Build history of the part. All positions in model axes, mm. Round coordinates to 2 decimals unless told otherwise and drop trailing zeros. Write each loop counter-clockwise with the first axis right and the second up, starting at its lowest first coordinate (ties: lowest second). Pieces come first, ordered by that corner, then holes. Notation, with made-up numbers: (27.25, 62) - (41.25, 62) arc R21 ccw to (41.25, 87) - close; hole circle Ø6 at (69.5, -23.75). An arc over 180 degrees is marked (long way). Answer as a JSON object with one key per item and string values. Group by question number.
Item 1: Probe line 1 (X direction, y = 0.4, z = -17) (3 decimals); line 2 (X direction, y = 0.7, z = 24.5). List the from-to ranges inside material, lowest first. Write a range as from..to.
Item 2: Slice it at B-B, the plane z = -8. List the corners of the cut face in (x, y) (3 decimals), then the cut area to 3 significant figures.
Item 3: Slice it at A-A, the plane y = 0.15. List the corners of the cut face in (x, z) (3 decimals), then the cut area to 3 significant figures.
Autodesk Inventor part; units mm, degrees
ref_plane "YZ Plane" through (0, 0, 0) normal (1, 0, 0) x (0, 1, 0)
ref_plane "XZ Plane" through (0, 0, 0) normal (0, 1, 0) x (-1, 0, 0)
ref_plane "XY Plane" through (0, 0, 0) normal (0, 0, 1) x (1, 0, 0)
sketch "Sketch1" plane through (0, 0, 0) normal (0, 1, 0) x (-1, 0, 0)
  line L0 (42.8, -26.99) -> (-42.8, -26.99)
  line L1 (-42.8, -26.99) -> (-42.8, 26.99)
  line L2 (-42.8, 26.99) -> (42.8, 26.99)
  line L3 (42.8, 26.99) -> (42.8, -26.99)
  line L4 (42.8, -26.99) -> (-42.8, 26.99) construction
  line L5 (-42.8, -26.99) -> (42.8, 26.99) construction
  point P0 (0, 0)
  dimension "d0" = 85.6
  dimension "d1" = 53.98
extrude "Extrusion1" add sketch "Sketch1" along normal blind 0.76
fillet "Fillet1" radius 2.88 4 edges at (42.8, 0.38, 26.99) (42.8, 0.38, -26.99) (-42.8, 0.38, 26.99) (-42.8, 0.38, -26.99)
sketch "Sketch2" plane through (0, 0, 0) normal (0, -1, 0) x (1, 0, 0)
  arc A0 (-42.8, -24.11) -> (-39.92, -26.99) centre (-39.92, -24.11) ccw
  line L0 (-39.92, -26.99) -> (39.92, -26.99)
  arc A1 (39.92, -26.99) -> (42.8, -24.11) centre (39.92, -24.11) ccw
  line L1 (42.8, -24.11) -> (42.8, 24.11)
  arc A2 (42.8, 24.11) -> (39.92, 26.99) centre (39.92, 24.11) ccw
  line L2 (39.92, 26.99) -> (-39.92, 26.99)
  arc A3 (-39.92, 26.99) -> (-42.8, 24.11) centre (-39.92, 24.11) ccw
  line L3 (-42.8, 24.11) -> (-42.8, -24.11)
  line L4 (-42.8, 24.11) -> (-42.8, -24.11)
  line L5 (-42.8, -3.99) -> (-39.625, -3.99)
  line L6 (-39.625, -3.99) -> (-39.625, -23.99)
  line L7 (-39.625, -23.99) -> (-42.8, -23.99)
  line L8 (-42.8, -23.99) -> (-42.8, -3.99)
  line L9 (42.8, 24.11) -> (42.8, -24.11)
  line L10 (42.8, -23.99) -> (39.625, -23.99)
  line L11 (39.625, -23.99) -> (39.625, -3.99)
  line L12 (39.625, -3.99) -> (42.8, -3.99)
  line L13 (42.8, -3.99) -> (42.8, -23.99)
  point P0 (0, 0)
  dimension "d5" = 3.175
  dimension "d6" = 3.175
  dimension "d7" = 3
  dimension "d8" = 3
  dimension "d9" = 20
  dimension "d10" = 20
extrude "Extrusion2" cut sketch "Sketch2" against normal through all contours L3 L5 L6 L7 | L10 L11 L12 L1
sketch "Sketch3" plane through (42.8, 0, 24.11) normal (1, 0, 0) x (0, 0, -1)
  line L0 (51.1, 0) -> (51.1, 0.76)
  line L1 (51.1, 0) -> (51.1, 0.76)
  line L2 (48.1, 0.76) -> (48.1, 0)
  line L3 (48.1, 0) -> (51.1, 0.76) construction
  line L4 (51.1, 0) -> (48.1, 0.76) construction
  line L5 (51.1, 0) -> (48.22, 0)
  arc A0 (48.1489, 0.76) -> (48.1489, 0) centre (49.6, 0.38) ccw
  arc A1 (51.0511, 0) -> (51.0511, 0.76) centre (49.6, 0.38) ccw
  line L6 (48.1, 0) -> (48.1489, 0)
  line L7 (51.0511, 0) -> (51.1, 0)
  line L8 (51.1, 0.76) -> (51.0511, 0.76)
  line L9 (48.1489, 0.76) -> (48.1, 0.76)
  point P0 (24.11, 0)
  point P1 (48.1, 0.38)
  point P2 (51.1, 0.38)
  dimension "d14" = 3
  dimension "d15" = 0.76
  dimension "d16" = 1.5
  dimension "d17" = 1.5
  dimension "d18" = 1.5
extrude "Extrusion3" cut sketch "Sketch3" against normal up to surface (3.175 mm away)
mirror "Mirror1" about plane through (0, 0, 0) normal (1, 0, 0) of "Extrusion3"
sketch "Sketch4" plane through (0, 0, 0) normal (0, -1, 0) x (1, 0, 0)
  line L0 (-39.625, -24.0389) -> (-42.8, -24.0389)
  line L1 (-42.8, -24.0389) -> (-42.8, -24.11)
  arc A0 (-42.8, -24.11) -> (-40.4486, -26.9411) centre (-39.92, -24.11) ccw
  line L2 (-40.4486, -26.9411) -> (-39.625, -26.9411)
  line L3 (-39.625, -26.9411) -> (-39.625, -26.99)
  line L4 (-39.625, -26.99) -> (39.625, -26.99)
  line L5 (39.625, -26.99) -> (39.625, -26.9411)
  line L6 (39.625, -26.9411) -> (40.4486, -26.9411)
  arc A1 (40.4486, -26.9411) -> (42.8, -24.11) centre (39.92, -24.11) ccw
  line L7 (42.8, -24.11) -> (42.8, -24.0389)
  line L8 (42.8, -24.0389) -> (39.625, -24.0389)
  line L9 (39.625, -24.0389) -> (39.625, -3.99)
  line L10 (39.625, -3.99) -> (42.8, -3.99)
  line L11 (42.8, -3.99) -> (42.8, 24.11)
  arc A2 (42.8, 24.11) -> (39.92, 26.99) centre (39.92, 24.11) ccw
  line L12 (39.92, 26.99) -> (-39.92, 26.99)
  arc A3 (-39.92, 26.99) -> (-42.8, 24.11) centre (-39.92, 24.11) ccw
  line L13 (-42.8, 24.11) -> (-42.8, -3.99)
  line L14 (-42.8, -3.99) -> (-39.625, -3.99)
  line L15 (-39.625, -3.99) -> (-39.625, -24.0389)
  line L16 (39.92, 26.99) -> (-39.92, 26.99)
  line L17 (42.8, -3.99) -> (42.8, 24.11)
  line L18 (-42.8, 24.11) -> (-42.8, -3.99)
  line L19 (-42.8, 26.99) -> (42.8, 26.99) construction
  line L20 (42.8, 26.99) -> (42.8, -27.0263) construction
  line L21 (42.8, -27.0263) -> (-42.8, -27.0263) construction
  line L22 (-42.8, -27.0263) -> (-42.8, 26.99) construction
  point P0 (0, 0)
decal "Decal1"
sketch "Sketch5" plane through (0, 0.76, 0) normal (0, 1, 0) x (1, 0, 0)
  line L0 (-42.8, 24.0389) -> (-39.625, 24.0389)
  line L1 (-39.625, 24.0389) -> (-39.625, 3.99)
  line L2 (-39.625, 3.99) -> (-42.8, 3.99)
  line L3 (-42.8, 3.99) -> (-42.8, -24.11)
  arc A0 (-42.8, -24.11) -> (-39.92, -26.99) centre (-39.92, -24.11) ccw
  line L4 (-39.92, -26.99) -> (39.92, -26.99)
  arc A1 (39.92, -26.99) -> (42.8, -24.11) centre (39.92, -24.11) ccw
  line L5 (42.8, -24.11) -> (42.8, 3.99)
  line L6 (42.8, 3.99) -> (39.625, 3.99)
  line L7 (39.625, 3.99) -> (39.625, 24.0389)
  line L8 (39.625, 24.0389) -> (42.8, 24.0389)
  line L9 (42.8, 24.0389) -> (42.8, 24.11)
  arc A2 (42.8, 24.11) -> (40.4486, 26.9411) centre (39.92, 24.11) ccw
  line L10 (40.4486, 26.9411) -> (39.625, 26.9411)
  line L11 (39.625, 26.9411) -> (39.625, 26.99)
  line L12 (39.625, 26.99) -> (-39.625, 26.99)
  line L13 (-39.625, 26.99) -> (-39.625, 26.9411)
  line L14 (-39.625, 26.9411) -> (-40.4486, 26.9411)
  arc A3 (-40.4486, 26.9411) -> (-42.8, 24.11) centre (-39.92, 24.11) ccw
  line L15 (-42.8, 24.11) -> (-42.8, 24.0389)
  line L16 (-42.8, 3.99) -> (-42.8, -24.11)
  line L17 (-42.8, 27.0263) -> (42.8, 27.0263) construction
  line L18 (42.8, 27.0263) -> (42.8, -26.99) construction
  line L19 (42.8, -26.99) -> (-42.8, -26.99) construction
  line L20 (-42.8, -26.99) -> (-42.8, 27.0263) construction
  line L21 (42.8, -24.11) -> (42.8, 3.99)
  point P0 (0, 0)
decal "Decal2"
equation "\"d0\" = cardWidth"
equation "\"d1\" = cardHeight"
equation "\"d2\" = cardThickness"
equation "\"d4\" = cardFillet"
equation "\"d5\" = materialThickness"
equation "\"d6\" = materialThickness"
equation "\"d7\" = cardPinDiameter"
equation "\"d8\" = cardPinDiameter"
equation "\"d9\" = cardCutoutHeight"
equation "\"d10\" = cardCutoutHeight"
equation "\"d11\" = cardThickness"
equation "\"d14\" = cardPinDiameter"
equation "\"d15\" = cardThickness"
equation "\"d16\" = 0.5 * cardPinDiameter"
equation "\"d18\" = 0.5 * cardPinDiameter"
equation "\"d19\" = cardThickness"
equation "\"materialThickness\" = 3.175"
equation "\"laserKerf\" = 0.12"
equation "\"cardPinDiameter\" = 3"
equation "\"centeralShaftDiameter\" = 8"
equation "\"cardWidth\" = 85.6"
equation "\"cardHeight\" = 53.98"
equation "\"cardThickness\" = 0.76"
equation "\"cardFillet\" = 2.88"
equation "\"cardCutoutHeight\" = 20"
equation "\"d13\" = cardPinDiameter"
equation "\"cardSelected\" = 1"
equation "\"cardClearence\" = 0.5"
equation "\"bearingOd\" = 22"
equation "\"bearingWidth\" = 8"
equation "\"axleHeight\" = 95"
equation "\"nutTrapDepth\" = 2.5"
equation "\"nutTrapwidth\" = 5.5"
equation "\"nutTrapClearence\" = 2"
equation "\"magnetLength\" = 3"
equation "\"magnetDiameter\" = 6"
equation "\"magnetProtusion\" = 0.25"
equation "\"spoolThickness\" = 5.588"
properties part number "card-01" material "ABS Plastic"
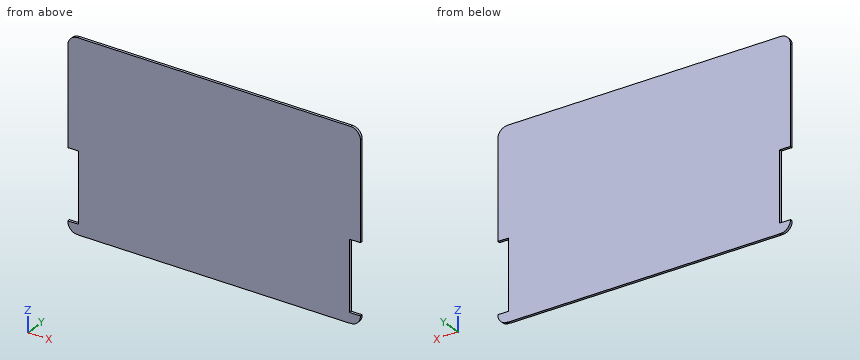
Geometry says:
{
 "1": {"line 1": "x = -39.625..39.625", "line 2": "x = -42.77..42.77"},
 "2": {"outline": "(-39.625, 0) - (39.625, 0) - (39.625, 0.76) - (-39.625, 0.76) - close", "area": "60.2 mm^2"},
 "3": {"outline": "(-42.8, -24.11) arc R2.88 ccw to (-40.239, -26.972) - (-39.625, -26.972) - (-39.625, -26.99) - (39.625, -26.99) - (39.625, -26.972) - (40.239, -26.972) arc R2.88 ccw to (42.8, -24.11) - (42.8, -24.008) - (39.625, -24.008) - (39.625, -3.99) - (42.8, -3.99) - (42.8, 24.11) arc R2.88 ccw to (39.92, 26.99) - (-39.92, 26.99) arc R2.88 ccw to (-42.8, 24.11) - (-42.8, -3.99) - (-39.625, -3.99) - (-39.625, -24.008) - (-42.8, -24.008) - close", "area": "4,490 mm^2"}
}
